CAD build for the part. Positions are in the model's coordinates, mm. Face numbers are marked on the shaded views. A direction names the side the tool comes from. Round coordinates to 2 decimals unless told otherwise and drop trailing zeros. Loops run counter-clockwise (first coordinate to the right, second up) from the corner with the lowest first, then second, coordinate; pieces in that order, holes last. Notation, with made-up numbers: M 69.25,0 L 80.25,0 A29 ccw 80.25,24 Z; hole C 43,54 d7. An arc over 180 degrees is marked long. Put each result on its own line as item: value. Start each with the question number.
from build123d import *

# Parameters (mm, degrees)
SKETCH_7_R      = 0.5
EXTRUDE_3_DEPTH = 5.7


with BuildPart() as part:
    # 草图7 → 凸台-拉伸3 (new body)
    with BuildSketch(Plane(origin=(0, 0, 0), x_dir=(0, 0, -1), z_dir=(1, 0, 0))):
        with BuildLine():
            ThreePointArc((-5.451006848, 0.732478218), (-4.945547363, 0.408928549), (-4.366855207, 0.249903181))
            ThreePointArc((-4.366855207, 0.249903181), (-4.374, 0), (-4.366855207, -0.249903181))
            ThreePointArc((-4.366855207, -0.249903181), (-4.945547363, -0.408928549), (-5.451006848, -0.732478218))
            ThreePointArc((-5.451006848, -0.732478218), (-5.432285873, -0.860389558), (-5.410563801, -0.987825571))
            ThreePointArc((-5.410563801, -0.987825571), (-4.829860918, -1.139344021), (-4.23035043, -1.111760422))
            ThreePointArc((-4.23035043, -1.111760422), (-4.159921202, -1.351640333), (-4.075901771, -1.58710452))
            ThreePointArc((-4.075901771, -1.58710452), (-4.577129176, -1.917172343), (-4.957867366, -2.381081934))
            ThreePointArc((-4.957867366, -2.381081934), (-4.900535883, -2.496947749), (-4.840497071, -2.61143411))
            ThreePointArc((-4.840497071, -2.61143411), (-4.241394034, -2.576089659), (-3.679749479, -2.364597169))
            ThreePointArc((-3.679749479, -2.364597169), (-3.538640333, -2.570972694), (-3.38597067, -2.76894901))
            ThreePointArc((-3.38597067, -2.76894901), (-3.760669693, -3.23774995), (-3.979417283, -3.796608762))
            ThreePointArc((-3.979417283, -3.796608762), (-3.889087297, -3.889087297), (-3.796608762, -3.979417283))
            ThreePointArc((-3.796608762, -3.979417283), (-3.23774995, -3.760669693), (-2.76894901, -3.38597067))
            ThreePointArc((-2.76894901, -3.38597067), (-2.570972694, -3.538640333), (-2.364597169, -3.679749479))
            ThreePointArc((-2.364597169, -3.679749479), (-2.576089659, -4.241394034), (-2.61143411, -4.840497071))
            ThreePointArc((-2.61143411, -4.840497071), (-2.496947749, -4.900535883), (-2.381081934, -4.957867366))
            ThreePointArc((-2.381081934, -4.957867366), (-1.917172343, -4.577129176), (-1.58710452, -4.075901771))
            ThreePointArc((-1.58710452, -4.075901771), (-1.351640333, -4.159921202), (-1.111760422, -4.23035043))
            ThreePointArc((-1.111760422, -4.23035043), (-1.139344021, -4.829860918), (-0.987825571, -5.410563801))
            ThreePointArc((-0.987825571, -5.410563801), (-0.860389558, -5.432285873), (-0.732478218, -5.451006848))
            ThreePointArc((-0.732478218, -5.451006848), (-0.408928549, -4.945547363), (-0.249903181, -4.366855207))
            ThreePointArc((-0.249903181, -4.366855207), (0, -4.374), (0.249903181, -4.366855207))
            ThreePointArc((0.249903181, -4.366855207), (0.408928549, -4.945547363), (0.732478218, -5.451006848))
            ThreePointArc((0.732478218, -5.451006848), (0.860389558, -5.432285873), (0.987825571, -5.410563801))
            ThreePointArc((0.987825571, -5.410563801), (1.139344021, -4.829860918), (1.111760422, -4.23035043))
            ThreePointArc((1.111760422, -4.23035043), (1.351640333, -4.159921202), (1.58710452, -4.075901771))
            ThreePointArc((1.58710452, -4.075901771), (1.917172343, -4.577129176), (2.381081934, -4.957867366))
            ThreePointArc((2.381081934, -4.957867366), (2.496947749, -4.900535883), (2.61143411, -4.840497071))
            ThreePointArc((2.61143411, -4.840497071), (2.576089659, -4.241394034), (2.364597169, -3.679749479))
            ThreePointArc((2.364597169, -3.679749479), (2.570972694, -3.538640333), (2.76894901, -3.38597067))
            ThreePointArc((2.76894901, -3.38597067), (3.23774995, -3.760669693), (3.796608762, -3.979417283))
            ThreePointArc((3.796608762, -3.979417283), (3.889087297, -3.889087297), (3.979417283, -3.796608762))
            ThreePointArc((3.979417283, -3.796608762), (3.760669693, -3.23774995), (3.38597067, -2.76894901))
            ThreePointArc((3.38597067, -2.76894901), (3.538640333, -2.570972694), (3.679749479, -2.364597169))
            ThreePointArc((3.679749479, -2.364597169), (4.241394034, -2.576089659), (4.840497071, -2.61143411))
            ThreePointArc((4.840497071, -2.61143411), (4.900535883, -2.496947749), (4.957867366, -2.381081934))
            ThreePointArc((4.957867366, -2.381081934), (4.577129176, -1.917172343), (4.075901771, -1.58710452))
            ThreePointArc((4.075901771, -1.58710452), (4.159921202, -1.351640333), (4.23035043, -1.111760422))
            ThreePointArc((4.23035043, -1.111760422), (4.829860918, -1.139344021), (5.410563801, -0.987825571))
            ThreePointArc((5.410563801, -0.987825571), (5.432285873, -0.860389558), (5.451006848, -0.732478218))
            ThreePointArc((5.451006848, -0.732478218), (4.945547363, -0.408928549), (4.366855207, -0.249903181))
            ThreePointArc((4.366855207, -0.249903181), (4.374, 0), (4.366855207, 0.249903181))
            ThreePointArc((4.366855207, 0.249903181), (4.945547363, 0.408928549), (5.451006848, 0.732478218))
            ThreePointArc((5.451006848, 0.732478218), (5.432285873, 0.860389558), (5.410563801, 0.987825571))
            ThreePointArc((5.410563801, 0.987825571), (4.829860918, 1.139344021), (4.23035043, 1.111760422))
            ThreePointArc((4.23035043, 1.111760422), (4.159921202, 1.351640333), (4.075901771, 1.58710452))
            ThreePointArc((4.075901771, 1.58710452), (4.577129176, 1.917172343), (4.957867366, 2.381081934))
            ThreePointArc((4.957867366, 2.381081934), (4.900535883, 2.496947749), (4.840497071, 2.61143411))
            ThreePointArc((4.840497071, 2.61143411), (4.241394034, 2.576089659), (3.679749479, 2.364597169))
            ThreePointArc((3.679749479, 2.364597169), (3.538640333, 2.570972694), (3.38597067, 2.76894901))
            ThreePointArc((3.38597067, 2.76894901), (3.760669693, 3.23774995), (3.979417283, 3.796608762))
            ThreePointArc((3.979417283, 3.796608762), (3.889087297, 3.889087297), (3.796608762, 3.979417283))
            ThreePointArc((3.796608762, 3.979417283), (3.23774995, 3.760669693), (2.76894901, 3.38597067))
            ThreePointArc((2.76894901, 3.38597067), (2.570972694, 3.538640333), (2.364597169, 3.679749479))
            ThreePointArc((2.364597169, 3.679749479), (2.576089659, 4.241394034), (2.61143411, 4.840497071))
            ThreePointArc((2.61143411, 4.840497071), (2.496947749, 4.900535883), (2.381081934, 4.957867366))
            ThreePointArc((2.381081934, 4.957867366), (1.917172343, 4.577129176), (1.58710452, 4.075901771))
            ThreePointArc((1.58710452, 4.075901771), (1.351640333, 4.159921202), (1.111760422, 4.23035043))
            ThreePointArc((1.111760422, 4.23035043), (1.139344021, 4.829860918), (0.987825571, 5.410563801))
            ThreePointArc((0.987825571, 5.410563801), (0.860389558, 5.432285873), (0.732478218, 5.451006848))
            ThreePointArc((0.732478218, 5.451006848), (0.408928549, 4.945547363), (0.249903181, 4.366855207))
            ThreePointArc((0.249903181, 4.366855207), (0, 4.374), (-0.249903181, 4.366855207))
            ThreePointArc((-0.249903181, 4.366855207), (-0.408928549, 4.945547363), (-0.732478218, 5.451006848))
            ThreePointArc((-0.732478218, 5.451006848), (-0.860389558, 5.432285873), (-0.987825571, 5.410563801))
            ThreePointArc((-0.987825571, 5.410563801), (-1.139344021, 4.829860918), (-1.111760422, 4.23035043))
            ThreePointArc((-1.111760422, 4.23035043), (-1.351640333, 4.159921202), (-1.58710452, 4.075901771))
            ThreePointArc((-1.58710452, 4.075901771), (-1.917172343, 4.577129176), (-2.381081934, 4.957867366))
            ThreePointArc((-2.381081934, 4.957867366), (-2.496947749, 4.900535883), (-2.61143411, 4.840497071))
            ThreePointArc((-2.61143411, 4.840497071), (-2.576089659, 4.241394034), (-2.364597169, 3.679749479))
            ThreePointArc((-2.364597169, 3.679749479), (-2.570972694, 3.538640333), (-2.76894901, 3.38597067))
            ThreePointArc((-2.76894901, 3.38597067), (-3.23774995, 3.760669693), (-3.796608762, 3.979417283))
            ThreePointArc((-3.796608762, 3.979417283), (-3.889087297, 3.889087297), (-3.979417283, 3.796608762))
            ThreePointArc((-3.979417283, 3.796608762), (-3.760669693, 3.23774995), (-3.38597067, 2.76894901))
            ThreePointArc((-3.38597067, 2.76894901), (-3.538640333, 2.570972694), (-3.679749479, 2.364597169))
            ThreePointArc((-3.679749479, 2.364597169), (-4.241394034, 2.576089659), (-4.840497071, 2.61143411))
            ThreePointArc((-4.840497071, 2.61143411), (-4.900535883, 2.496947749), (-4.957867366, 2.381081934))
            ThreePointArc((-4.957867366, 2.381081934), (-4.577129176, 1.917172343), (-4.075901771, 1.58710452))
            ThreePointArc((-4.075901771, 1.58710452), (-4.159921202, 1.351640333), (-4.23035043, 1.111760422))
            ThreePointArc((-4.23035043, 1.111760422), (-4.829860918, 1.139344021), (-5.410563801, 0.987825571))
            ThreePointArc((-5.410563801, 0.987825571), (-5.432285873, 0.860389558), (-5.451006848, 0.732478218))
        make_face()
        with Locations((0, 2.76894901)):
            Circle(SKETCH_7_R, mode=Mode.SUBTRACT)
        with BuildLine():
            Line((0.442162115, -0.896935151), (0.442162115, 0.896935151))
            ThreePointArc((0.442162115, 0.896935151), (-1, 0), (0.442162115, -0.896935151))
        make_face(mode=Mode.SUBTRACT)
    extrude(amount=EXTRUDE_3_DEPTH)


solid = part.part
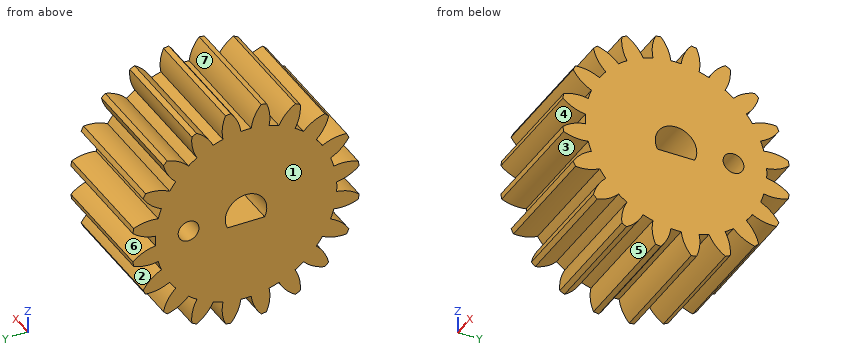
(1) Flat gauge pins, fed straight in: pin 1 Ø1.8 at (y, z) = (0, 0) entering from -X; pin 2 Ø1.5 at (x, y) = (2.5, -2.5) entering from +Z; pin 3 Ø1.5 at (x, z) = (2, 2.5) entering from +Y; pin 4 Ø1.4 at (x, y) = (1.5, 0) entering from +Z. Where does each tip first touch, or does it go through?
(2) Cut at B-B on z = 0. List the corners of the cut face in (x, y).
(3) Cut at C-C on y = 3. List the corners of the cut face in (x, z).
(4) Drill centre lines: line 1 along Z through (x, y) = (4.35, 4.75); line 2 along Y through (x, z) = (1.4, 4.5). Where is each one in solid material? Low to high.
(5) Cut at D-D on x = 4.2. Count the separate pieces of the cut face and the enclosed holes in it, and give its area (3 significant figures).
(6) Mould opens along Y. For the marked faces 1, 2 and 3 say: +Y half, -Y half, draft (parallel to the pull), parting line (faces both ways), or undercut.
(7) Cut at A-A on y = 0. List the corners of the cut face in (x, z).
(8) Tool access for the marked faces 4, 5, 6 and 7: list every direction of +Z, -Z, +X, -X, +Y, -Y with a clear straight run to the whole face (end or side of a thin tool).
Taken from the geometry:
1. pin 1: x = 0
1. pin 2: z = 4.96
1. pin 3: y = 4.96
1. pin 4: z = 5.41
2. outline: M 0,-4.37 L 5.7,-4.37 L 5.7,-1 L 0,-1 Z; M 0,1 L 5.7,1 L 5.7,2.27 L 0,2.27 Z; M 0,3.27 L 5.7,3.27 L 5.7,4.37 L 0,4.37 Z
3. outline: M 0,-3.6 L 5.7,-3.6 L 5.7,-0.44 L 0,-0.44 Z; M 0,0.44 L 5.7,0.44 L 5.7,3.6 L 0,3.6 Z
4. line 1: -2.62 to -2.09, -1.15 to -0.33, 0.33 to 1.15, 2.09 to 2.62
4. line 2: -2.61 to -1.85, -1.15 to -0.27, 0.27 to 1.15, 1.85 to 2.61
5. separate pieces: 1
5. enclosed holes: 2
5. area: 72.5 mm2
6. face 1: draft
6. face 2: +Y half
6. face 3: undercut
7. outline: M 0,-4.37 L 5.7,-4.37 L 5.7,-0.44 L 0,-0.44 Z; M 0,1 L 5.7,1 L 5.7,4.37 L 0,4.37 Z
8. face 4: +X, -X, -Y
8. face 5: +X, -X
8. face 6: +X, -X, +Y
8. face 7: +Z, +X, -X
